Could you check a few things on this model? Use its own coordinates, in mm. A direction names the side the tool comes from. Coordinates: 2 decimals unless noted, no trailing zeros. Write each loop counter-clockwise with the first axis right and the second up, starting at its lowest first coordinate (ties: lowest second). Pieces come first, ordered by that corner, then holes.
```python
from build123d import *

# Parameters (mm, degrees)
F0_W     = 100
F0_H     = 100
F0_R     = 25
F1_DEPTH = 100
F2_W     = 80
F2_H     = 100
F3_DEPTH = 100
F4_R     = 5
F5_DEPTH = 100


with BuildPart() as f1:
    # F0 (on Top) → F1 (new body)
    with BuildSketch(Plane.XY):
        Rectangle(F0_W, F0_H)
        Circle(F0_R, mode=Mode.SUBTRACT)
    extrude(amount=F1_DEPTH)

    # F2 (on face) → F3 (cut)
    with BuildSketch(Plane.YZ.offset(50)):
        Rectangle(F2_W, F2_H)
    extrude(amount=-F3_DEPTH, mode=Mode.SUBTRACT)

    # F4 (on face) → F5 (cut)
    with BuildSketch(Plane(origin=(0, 50, 0), x_dir=(-1, 0, 0), z_dir=(0, 1, 0))):
        with Locations((0, 20)):
            Circle(F4_R)
    extrude(amount=-F5_DEPTH, mode=Mode.SUBTRACT)


solid = f1.part
```
1. I want a section at D-D on z = 20. Please give me the cut outline in (x, y), plus the area to 3 significant figures.
Verdict:
outline: (-50, -50) - (-5, -50) - (-5, -40) - (-50, -40) - close; (-50, 40) - (-5, 40) - (-5, 50) - (-50, 50) - close; (5, -50) - (50, -50) - (50, -40) - (5, -40) - close; (5, 40) - (50, 40) - (50, 50) - (5, 50) - close
area: 1,800 mm2
2. I want a section at B-B on z = 8.5. Please give me the cut outline in (x, y), plus the area to 3 significant figures.
Verdict:
outline: (-50, -50) - (50, -50) - (50, -40) - (-50, -40) - close; (-50, 40) - (50, 40) - (50, 50) - (-50, 50) - close
area: 2,000 mm2
3. I want a section at C-C on y = 0. Please give me the cut outline in (x, z), plus the area to 3 significant figures.
Verdict:
outline: (-50, 50) - (-25, 50) - (-25, 100) - (-50, 100) - close; (25, 50) - (50, 50) - (50, 100) - (25, 100) - close
area: 2,500 mm2
4. I want a section at A-A on x = 0. Please give me the cut outline in (y, z).
Verdict:
outline: (-50, 0) - (-40, 0) - (-40, 15) - (-50, 15) - close; (-50, 25) - (-40, 25) - (-40, 50) - (-25, 50) - (-25, 100) - (-50, 100) - close; (25, 50) - (40, 50) - (40, 25) - (50, 25) - (50, 100) - (25, 100) - close; (40, 0) - (50, 0) - (50, 15) - (40, 15) - close
5. On a 3-axis mill with a long thin cutter (end or side, diameter ignored), from which of +Z, -Z, +X, -X, +Y, -Y can I reach the whole of each face in a straight line? I mean faces 1 (the face through (1, -40, 30)), 2 (the face through (-1, -45, 0)). Say none if no direction works.
Verdict:
face 1: -Z, +X, -X
face 2: -Z, +X, -X, +Y, -Y
6. If we mould it in two halves opening along X, with no side actions, what happens to faces 3 (the face through (-50, -1, 72)), 4 (the face through (-1, 45, 0)), 5 (the face through (23.846, 7.509, 74.65))? For each: pulls with the +X half, pulls with the -X half, needs draft (parallel to the pull), parting line crosses it, or undercut.
Verdict:
face 3: pulls with the -X half
face 4: needs draft
face 5: undercut
7. Please list where these lines run through material, in increasing order: line 1 along Y through (x, z) = (0, 89.5); line 2 along Y through (x, z) = (9, 37.5); line 3 along Z through (x, y) = (0, 46.75).
Verdict:
line 1: y = -50 to -25, 25 to 50
line 2: y = -50 to -40, 40 to 50
line 3: z = 0 to 15, 25 to 100
